Input: part model. Units: mm. Frame: model coordinates. Face numbers are marked on the shaded views. A direction names the side the tool comes from. Give positions to 0.01 mm unless a question says otherwise; leave off trailing zeros. Write each loop counter-clockwise with the first axis right and the second up, starting at its lowest first coordinate (ties: lowest second). Pieces come first, ordered by that corner, then holes. Notation, with made-up numbers: M 70,42 L 101,42 A30 cw 101,69 Z; hole C 11.5,-10 d11. An arc over 180 degrees is marked long. Use CSV: the item, a comma, the result in double quotes. Start each with the question number.
from build123d import *

# Parameters (mm, degrees)
BOSS_EXTRUDE1_DEPTH = 17
FILLET1_R           = 0.3
FILLET2_R           = 0.2
SKETCH2_W           = 2.1
SKETCH2_H           = 0.2
TAPPED_HOLE1_D      = 4.134


with BuildPart() as part:
    # Sketch1 → Boss-Extrude1 (new body)
    with BuildSketch(Plane(origin=(-6, 0, 0), x_dir=(0, 0, -1), z_dir=(1, 0, 0))):
        with BuildLine():
            Line((2.9, 0), (-2.9, 0))
            Line((-2.9, 0), (-2.9, -0.7))
            Line((-2.9, -0.7), (-3.95, -0.7))
            ThreePointArc((-3.95, -0.7), (-4.13076842, -0.814426765), (-4.104689384, -1.026772215))
            Line((-4.104689384, -1.026772215), (-1.75, -3.9))
            Line((-1.75, -3.9), (1.75, -3.9))
            Line((1.75, -3.9), (4.104689384, -1.026772215))
            ThreePointArc((4.104689384, -1.026772215), (4.13076842, -0.814426765), (3.95, -0.7))
            Line((3.95, -0.7), (2.9, -0.7))
            Line((2.9, -0.7), (2.9, 0))
        make_face()
    extrude(amount=BOSS_EXTRUDE1_DEPTH)

    # Fillet1
    fillet1_edges = [part.edges().sort_by_distance(p)[0] for p in [
        (2.5, -3.9, -1.75),
        (2.5, -3.9, 1.75),
    ]]
    fillet(fillet1_edges, radius=FILLET1_R)

    # Fillet2
    fillet2_edges = [part.edges().sort_by_distance(p)[0] for p in [
        (2.5, 0, 2.9),
        (2.5, 0, -2.9),
    ]]
    fillet(fillet2_edges, radius=FILLET2_R)

    # Sketch2 → Cut-Revolve1 (revolve, cut)
    with BuildSketch(Plane(origin=(7.5, 0, 0), x_dir=(0, 0, -1), z_dir=(1, 0, 0))):
        with Locations((1.05, -3.8)):
            Rectangle(SKETCH2_W, SKETCH2_H)
    revolve(axis=Axis((7.5, 1.665548573, 0), (0, -1, 0)), mode=Mode.SUBTRACT)

    # Sketch3 → Revolve1 (revolve)
    with BuildSketch(Plane(origin=(7.5, 0, 0), x_dir=(0, 0, -1), z_dir=(1, 0, 0))):
        with BuildLine():
            Line((1.732050808, -3.7), (0, -3.7))
            Line((0, -3.7), (0, -4.7))
            ThreePointArc((0, -4.7), (1, -4.432050808), (1.732050808, -3.7))
        make_face()
    revolve(axis=Axis((7.5, 0, 0), (0, -1, 0)))

    # Tapped Hole1 (through all)
    with Locations(Plane(origin=(0, 0, 0), x_dir=(1, 0, 0), z_dir=(0, 1, 0))):
        with Locations((0, 0)):
            Hole(TAPPED_HOLE1_D / 2)


solid = part.part
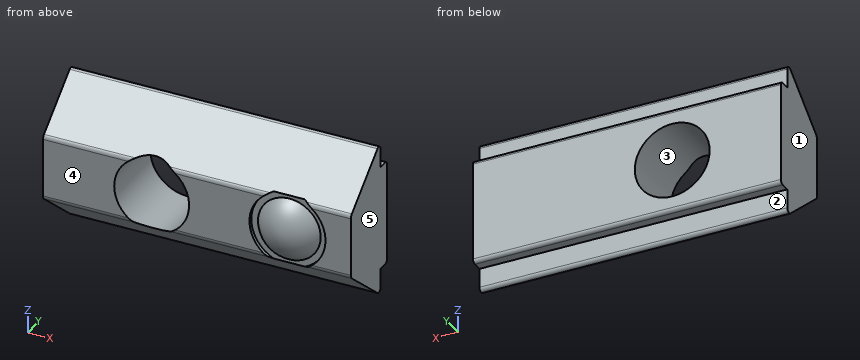
Q1. Section C-C, the plane y = -2.7. Return the cut outline in (x, z), and give its area (3 significant figures).
Q2. Section B-B, the plane x = 0. Return the cut outline in (y, z).
Q3. Pull-direction query (X, two-part tool) for the marked faces 3, 4 and 5; classes: released by +X, released by -X, zero draft, split by the parting line, or undercut.
Q4. Section D-D, the plane x = -4.25. Return the cut outline in (y, z), and give its area (3 significant figures).
Q5. Set-up query: the marked faces 1 and 2. Return all of +Z, -Z, +X, -X, +Y, -Y with unobstructed straight access to the full face (end or side cutting, diameter ignored); none if empty.
Q6. Section A-A, the plane z = 0. Return the cut outline in (x, y).
Q7. First-contact query: pin 1 Ø0.5 at (x, z) = (4.5, -3.5) entering from +Y; pin 2 Ø1.1 at (x, z) = (7, 0.5) entering from -Y; pin 3 Ø1.6 at (x, z) = (-4, -0.5) entering from -Y. Flat tips, straight axial feed; report the tip coordinate or a pass-through.
Q8. Material intervals for L1, parallel to Y at x = 7.5, z = -1.75; L2, parallel to X at y = -2.7, z = -0.5; L3, parallel to Z at x = 0, y = -3, sorted ascending. Write a range as [from, to].
Check result:
1,outline,"M -6,-2.73 L 11,-2.73 L 11,2.73 L -6,2.73 Z; hole C 0,0 d4.13"
1,area,"79.5 mm²"
2,outline,"M -3.51,-2.07 L -1.03,-4.1 A0.2 ccw -0.7,-3.95 L -0.7,-2.9 L -0.2,-2.9 A0.2 ccw 0,-2.7 L 0,-2.07 Z; M -3.51,2.07 L 0,2.07 L 0,2.7 A0.2 ccw -0.2,2.9 L -0.7,2.9 L -0.7,3.95 A0.2 ccw -1.03,4.1 Z"
3,face 3,"undercut"
3,face 4,"zero draft"
3,face 5,"released by +X"
4,outline,"M -3.9,-1.61 A0.3 ccw -3.79,-1.84 L -1.03,-4.1 A0.2 ccw -0.7,-3.95 L -0.7,-2.9 L -0.2,-2.9 A0.2 ccw 0,-2.7 L 0,2.7 A0.2 ccw -0.2,2.9 L -0.7,2.9 L -0.7,3.95 A0.2 ccw -1.03,4.1 L -3.79,1.84 A0.3 ccw -3.9,1.61 Z"
4,area,"23.6 mm²"
5,face 1,"+Z, -Z, -X, +Y, -Y"
5,face 2,"-Z, +X, -X, +Y"
6,outline,"M -6,-3.9 L -2.07,-3.9 L -2.07,0 L -6,0 Z; M 2.07,-3.9 L 5.4,-3.9 L 5.4,-3.7 L 5.77,-3.7 A2 ccw 9.23,-3.7 L 9.6,-3.7 L 9.6,-3.9 L 11,-3.9 L 11,0 L 2.07,0 Z"
7,pin 1,"stops at y = -0.7"
7,pin 2,"stops at y = -4.69"
7,pin 3,"stops at y = -3.9"
8,L1,"y = [-3.7, 0]"
8,L2,"x = [-6, -2.01], [2.01, 11]"
8,L3,"z = [-2.49, -2.07], [2.07, 2.49]"
